from build123d import *

# Parameters (mm, degrees)
BOSS_EXTRUDE1_DEPTH = 72
SKETCH2_R           = 4.25
CUT_EXTRUDE1_DEPTH  = 65
SKETCH3_R           = 6.35
BOSS_EXTRUDE2_DEPTH = 26
SKETCH5_R           = 6.35
BOSS_EXTRUDE3_DEPTH = 26


with BuildPart() as part:
    # Sketch1 → Boss-Extrude1 (new body)
    with BuildSketch(Plane.XY):
        Polygon((-56.490044248, 32.210989011), (58.009955752, 32.210989011), (70, 32.210989011), (70, 26.210989011), (55.75, 26.210989011), (55.75, -31.789010989), (-57.25, -31.789010989), (-57.25, 26.210989011), (-70, 26.210989011), (-70, 32.210989011), align=None)
    extrude(amount=BOSS_EXTRUDE1_DEPTH)

    # Sketch2 → Cut-Extrude1 (cut, through all)
    with BuildSketch(Plane(origin=(0, 32.210989011, 0), x_dir=(1, 0, 0), z_dir=(0, 1, 0))):
        with Locations((61.5, -36)):
            Circle(SKETCH2_R)
        with BuildLine():
            Line((-61.5, -31.5), (-70, -31.5))
            Line((-70, -31.5), (-70, -40.5))
            Line((-70, -40.5), (-61.5, -40.5))
            ThreePointArc((-61.5, -40.5), (-57, -36), (-61.5, -31.5))
        make_face()
    extrude(amount=-CUT_EXTRUDE1_DEPTH, mode=Mode.SUBTRACT)

    # Sketch3 → Boss-Extrude2 (add)
    with BuildSketch(Plane.XY.offset(72)):
        Circle(SKETCH3_R)
    extrude(amount=BOSS_EXTRUDE2_DEPTH)

    # Sketch5 → Boss-Extrude3 (add)
    with BuildSketch(Plane(origin=(0, 0, 0), x_dir=(-1, 0, 0), z_dir=(0, 0, -1))):
        Circle(SKETCH5_R)
    extrude(amount=BOSS_EXTRUDE3_DEPTH)


solid = part.part
CAD build for the part. Positions are in the model's coordinates, mm. A direction names the side the tool comes from. Give positions to 0.01 mm unless a question says otherwise; leave off trailing zeros. Order: outer loops, then holes, each group sorted by start corner. A loop starts at its lowest first (then second) coordinate and runs counter-clockwise, first axis right, second up. Notation, with made-up numbers: (-6.5, 86.5) - (30.5, 86.5) arc R29 cw to (30.5, 115.5) - close; hole circle Ø8 at (61, 55). An arc over 180 degrees is marked (long way). Answer in a Markdown table with one row per item.
1. Pull direction Z, two halves, no side cores. Call faces 1 (the cylindrical face through (-57, 7, 36)), 2 (the flat face through (1, 8, 0)), 3 (the flat face through (-57.25, -3, 17)): pulls with the +Z half, pulls with the -Z half, needs draft (parallel to the pull), parting line crosses it, or undercut.
Data:
| item | result |
|---|---|
| face 1 | undercut |
| face 2 | pulls with the -Z half |
| face 3 | needs draft |
2. Probe probe 1 along X at (y, z) = (28, 36); probe 2 along Z at (x, y) = (61, 30); probe 3 along Z at (x, y) = (-19, 15.5). List the from-to ranges inside material, lowest first. Write a range as [from, to].
Data:
| item | result |
|---|---|
| probe 1 | x = [-57, 57.25], [65.75, 70] |
| probe 2 | z = [0, 31.78], [40.22, 72] |
| probe 3 | z = [0, 72] |
3. Flat gauge pins, fed straight in: pin 1 (19 mm diameter, centred on x = 11.5, y = -6.5, fed in from -Z); pin 2 (7.5 mm diameter, centred on x = 61.5, z = 36, fed in from +Y); pin 3 (2 mm diameter, centred on y = 2, z = 11.5, fed in from -X); pin 4 (6.5 mm diameter, centred on x = -64, y = 28.5, fed in from +Z). Where does each tip first touch, or does it go through?
Data:
| item | result |
|---|---|
| pin 1 | stops at z = -26 |
| pin 2 | passes through |
| pin 3 | stops at x = -57.25 |
| pin 4 | stops at z = 72 |
4. Saw through at D-D, the plane x = 0. Give the cut face in (y, z), plus the area to 3 significant figures.
Data:
| item | result |
|---|---|
| outline | (-31.79, 0) - (-6.35, 0) - (-6.35, -26) - (6.35, -26) - (6.35, 0) - (32.21, 0) - (32.21, 72) - (6.35, 72) - (6.35, 98) - (-6.35, 98) - (-6.35, 72) - (-31.79, 72) - close |
| area | 5,270 mm² |
5. Saw through at B-B, the plane z = 3.5. Give the cut face in (x, y).
Data:
| item | result |
|---|---|
| outline | (-70, 26.21) - (-57.25, 26.21) - (-57.25, -31.79) - (55.75, -31.79) - (55.75, 26.21) - (70, 26.21) - (70, 32.21) - (-70, 32.21) - close |
6. Saw through at C-C, the plane y = 0. Give the cut face in (x, z).
Data:
| item | result |
|---|---|
| outline | (-57.25, 0) - (-6.35, 0) - (-6.35, -26) - (6.35, -26) - (6.35, 0) - (55.75, 0) - (55.75, 72) - (6.35, 72) - (6.35, 98) - (-6.35, 98) - (-6.35, 72) - (-57.25, 72) - (-57.25, 37.48) arc R4.5 cw to (-57.25, 34.52) - close |
7. Tool access for faces 4 (the flat face through (-64, 26.211, 54)), 5 (the flat face through (55.75, -2, 35)), 6 (the flat face through (-66, 29, 40.5)), 7 (the cylindrical face through (-1.38, -6.2, 84.82)): list every direction of +Z, -Z, +X, -X, +Y, -Y with a clear straight run to the whole face (end or side of a thin tool).
Data:
| item | result |
|---|---|
| face 4 | +Z, -Z, -X, -Y |
| face 5 | +Z, -Z, +X, -Y |
| face 6 | -X, +Y, -Y |
| face 7 | +Z |
8. Saw through at A-A, the plane x = 61.5. Give the cut face in (y, z), plus the area to 3 significant figures.
Data:
| item | result |
|---|---|
| outline | (26.21, 0) - (32.21, 0) - (32.21, 31.75) - (26.21, 31.75) - close; (26.21, 40.25) - (32.21, 40.25) - (32.21, 72) - (26.21, 72) - close |
| area | 381 mm² |
